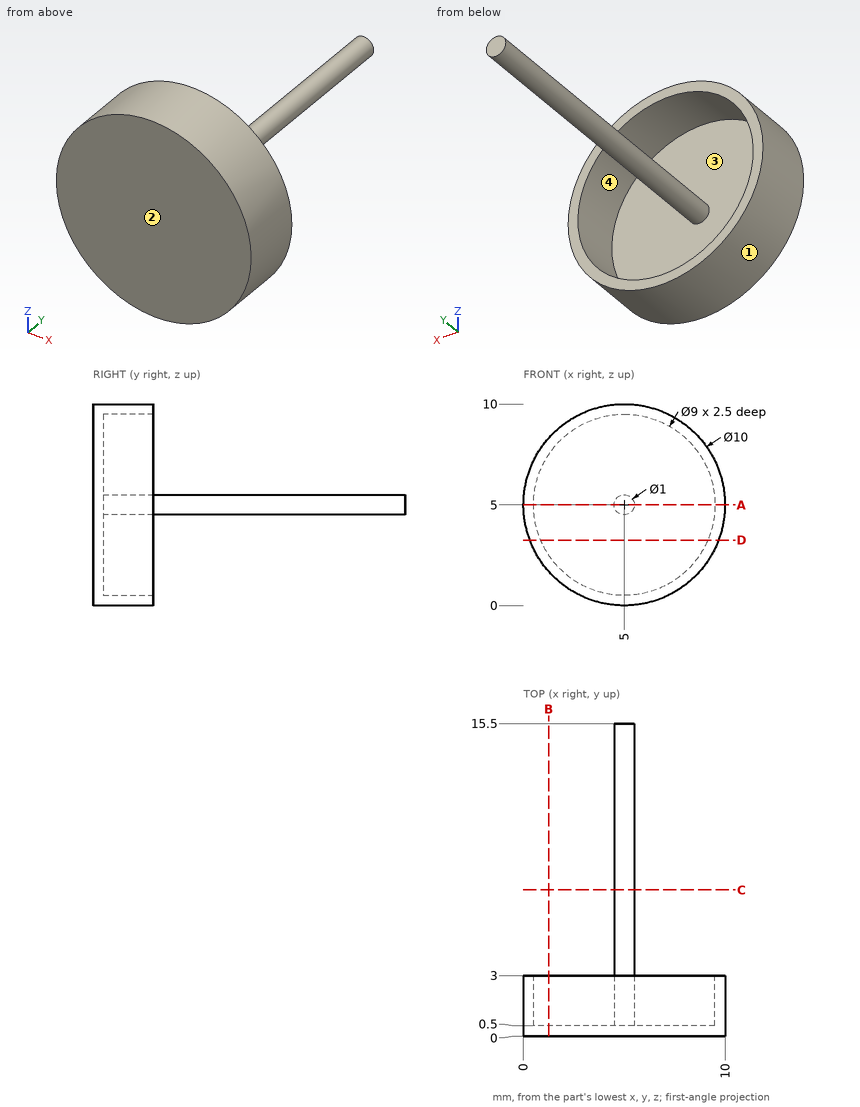
Drawing for the job (mm, zero at the part's lowest x, y, z). Give positions to 0.01 mm unless a question says otherwise; leave off trailing zeros. Write each loop counter-clockwise with the first axis right and the second up, starting at its lowest first coordinate (ties: lowest second). Pieces come first, ordered by that corner, then holes. Notation, with made-up numbers: (5, -14) -> (10, -14) arc R10 cw to (10, -6) -> close; hole circle Ø7 at (89, 62). An arc over 180 degrees is marked (long way). Put each result on its own line as item: value. Start each with the question number.
Item 1: Pin check, flat tips, straight feed: pin 1 Ø6 at (y, z) = (4.5, 2.5) entering from +X; pin 2 Ø1.5 at (x, z) = (6.5, 2.5) entering from +Y; pin 3 Ø5 at (y, z) = (7.5, 2.5) entering from -X; pin 4 Ø1.5 at (y, z) = (3.5, 2.5) entering from +X. Stop position of each tip, or through.
Item 2: Wall check: L1, parallel to X at y = 1.7, z = 5; L2, parallel to Y at x = 1, z = 5.5; L3, parallel to Y at x = 2.75, z = 0.75. Give the ranges that are in metal, low to high. Write a range as [from, to].
Item 3: Cut at A-A (z = 5). List the corners of the cut face in (x, y).
Item 4: Cut at B-B (x = 1.25). List the corners of the cut face in (y, z), then the cut area to 3 significant figures.
Item 5: Pull direction X, two halves, no side cores. Call the marked faces 1, 2, 3 and 4: pulls with the +X half, pulls with the -X half, needs draft (parallel to the pull), parting line crosses it, or undercut.
Item 6: Cut at D-D (z = 3.25). List the corners of the cut face in (x, y), then the cut area to 3 significant figures.
Item 7: Cut at C-C (y = 7.25). List the corners of the cut face in (x, z), then the cut area to 3 significant figures.
Answer list:
1. pin 1: stops at x = 10
1. pin 2: stops at y = 0.5
1. pin 3: stops at x = 4.5
1. pin 4: stops at x = 9.61
2. L1: x = [0, 0.5], [4.5, 5.5], [9.5, 10]
2. L2: y = [0, 0.5]
2. L3: y = [0, 3]
3. outline: (0, 0) -> (10, 0) -> (10, 3) -> (9.5, 3) -> (9.5, 0.5) -> (5.5, 0.5) -> (5.5, 15.5) -> (4.5, 15.5) -> (4.5, 0.5) -> (0.5, 0.5) -> (0.5, 3) -> (0, 3) -> close
4. outline: (0, 1.69) -> (3, 1.69) -> (3, 2.51) -> (0.5, 2.51) -> (0.5, 7.49) -> (3, 7.49) -> (3, 8.31) -> (0, 8.31) -> close
4. area: 7.41 mm2
5. face 1: parting line crosses it
5. face 2: needs draft
5. face 3: undercut
5. face 4: undercut
6. outline: (0.32, 0) -> (9.68, 0) -> (9.68, 3) -> (9.15, 3) -> (9.15, 0.5) -> (0.85, 0.5) -> (0.85, 3) -> (0.32, 3) -> close
6. area: 7.37 mm2
7. outline: circle Ø1 at (5, 5)
7. area: 0.785 mm2
